Solid Edge part; units mm, degrees
sketch "Sketch1" plane through (0, 0, 0) normal (0, -1, 0) x (1, 0, 0)
  line L0 (-8.5, -24) -> (8.5, -24)
  line L1 (8.5, -24) -> (8.5, 24)
  line L2 (8.5, 24) -> (-8.5, 24)
  line L3 (-8.5, 24) -> (-8.5, -24)
  dimension "D1" = 8.5
  dimension "D2" = 8.5
extrude "Protrusion1" add sketch "Sketch1" along normal mid plane 5
sketch "Sketch2" plane through (0, -2.5, 0) normal (0, -1, 0) x (1, 0, 0)
  circle A0 centre (0, 15.56) radius 6.5
extrude "Extrusionsausschnitt_1" cut sketch "Sketch2" against normal blind 64
hole "Bohrung_1" at (-5, 0, -24) direction (0, 0, 1) diameter 3.5 depth 8
hole "Hole1" at (5, 0, -24) direction (0, 0, 1) diameter 3.5 depth 8
sketch "Sketch3" plane through (0, 0, 24) normal (0, 0, 1) x (1, 0, 0)
  line L0 (-8.5, 2.5) -> (8.5, 2.5)
  line L1 (8.5, 2.5) -> (8.5, -2.5)
  line L2 (8.5, -2.5) -> (-8.5, -2.5)
  line L3 (-8.5, -2.5) -> (-8.5, 2.5)
extrude "Extrusionsausprägung_2" add sketch "Sketch3" along normal blind 6
hole "Bohrung_5" at (-5, 0, 30) direction (0, 0, -1) diameter 3.5 depth 8
hole "Hole2" at (5, 0, 30) direction (0, 0, -1) diameter 3.5 depth 8
properties material "Aluminiumlegierung:3.0205, Al 99.0, EN-AW 1200"
The model under review builds one solid part; all positions refer to its coordinate system, in mm. A direction names the side the tool comes from. Round coordinates to 2 decimals unless told otherwise and drop trailing zeros. Loops run counter-clockwise (first coordinate to the right, second up) from the corner with the lowest first, then second, coordinate; pieces in that order, holes last. Notation, with made-up numbers: (66.25, -24) - (74.25, -24) arc R13 ccw to (74.25, -9) - close; hole circle Ø3 at (-7, -35.75). An arc over 180 degrees is marked (long way). Use CSV: the item, a comma, the result in double quotes.
(1) Machinability: for faces 1 (the flat face through (-5, 0, 22)), 2 (the flat face through (-5, 0, -16)), 3 (the flat face through (8.5, 0, 3)), which of the approach directions +Z, -Z, +X, -X, +Y, -Y give a long, thin tool a straight path to every point of the face, cutting with its end or side? Answer none if there is none.
Working result:
face 1,"+Z"
face 2,"-Z"
face 3,"+Z, -Z, +X, +Y, -Y"
(2) The part is to be moulded in two halves that separate along Y. For faces 4 (the cylindrical face through (-0.846, -0.035, 22.005)), 5 (the cylindrical face through (6.71, -0.38, -19.94)), 6 (the flat face through (0, 2.5, 3)), 7 (the flat face through (5, 0, 22)), say which applies: pulls with the +Y half, pulls with the -Y half, needs draft (parallel to the pull), parting line crosses it, or undercut.
Working result:
face 4,"needs draft"
face 5,"undercut"
face 6,"pulls with the +Y half"
face 7,"undercut"
(3) Take a section at A-A, the plane x = 0. Give the boundary of the cut face in (y, z), plus the area to 3 significant figures.
Working result:
outline,"(-2.5, -24) - (2.5, -24) - (2.5, 9.06) - (-2.5, 9.06) - close; (-2.5, 22.06) - (2.5, 22.06) - (2.5, 30) - (-2.5, 30) - close"
area,"205 mm^2"
(4) Take a section at B-B, the plane z = 21. Give the boundary of the cut face in (x, y).
Working result:
outline,"(-8.5, -2.5) - (-3.56, -2.5) - (-3.56, 2.5) - (-8.5, 2.5) - close; (3.56, -2.5) - (8.5, -2.5) - (8.5, 2.5) - (3.56, 2.5) - close"
(5) For line 1 (X direction, y = 0, z = -17.75); line 2 (Z direction, x = 0, y = 0.55); line 3 (Y direction, x = 5, z = 26), list the stretches that pass through material, from the lowest coordinate up.
Working result:
line 1,"x = -8.5 to -6.75, -3.25 to 3.25, 6.75 to 8.5"
line 2,"z = -24 to 9.06, 22.06 to 30"
line 3,"y = -2.5 to -1.75, 1.75 to 2.5"
(6) Take a section at D-D, the plane x = -5. Give the boundary of the cut face in (y, z), plus the area to 3 significant figures.
Working result:
outline,"(-2.5, -24) - (-1.75, -24) - (-1.75, -16) - (1.75, -16) - (1.75, -24) - (2.5, -24) - (2.5, 11.41) - (-2.5, 11.41) - close; (-2.5, 19.71) - (2.5, 19.71) - (2.5, 30) - (1.75, 30) - (1.75, 22) - (-1.75, 22) - (-1.75, 30) - (-2.5, 30) - close"
area,"172 mm^2"
(7) Clearance check with flat-ended pins moving along their axes: P1, Ø3, axis at x = 5, y = 0, coming from the +Z side; P2, Ø1, axis at x = -5, y = 1, coming from the -Z side. State where each tip first meets the part, or that it passes through.
Working result:
P1,"stops at z = 22"
P2,"stops at z = -16"
(8) Take a section at C-C, the plane y = 0. Give the boundary of the cut face in (x, z), plus the area to 3 significant figures.
Working result:
outline,"(-8.5, -24) - (-6.75, -24) - (-6.75, -16) - (-3.25, -16) - (-3.25, -24) - (3.25, -24) - (3.25, -16) - (6.75, -16) - (6.75, -24) - (8.5, -24) - (8.5, 30) - (6.75, 30) - (6.75, 22) - (3.25, 22) - (3.25, 30) - (-3.25, 30) - (-3.25, 22) - (-6.75, 22) - (-6.75, 30) - (-8.5, 30) - close; hole circle Ø13 at (0, 15.56)"
area,"673 mm^2"
